from build123d import *

# Parameters (mm, degrees)
F3_W = 25.4
F3_H = 50.8
F5_R = 6.35


with BuildPart() as f4:
    # F4: sweep along a path in F1
    with BuildLine(Plane.XZ) as f4_path:
        Line((4636.6553444, 766.7224442), (5169.5693154, 766.7224442))
        Line((5169.5693154, 766.7224442), (5169.5693154, -249.2775558))
        Line((5169.5693154, -249.2775558), (4636.6553444, -249.2775558))
    # F3 (on plane+point) → F4 (sweep)
    with BuildSketch(Plane.YZ.offset(4636.6553444)):
        with Locations((0, 766.7224442)):
            Rectangle(F3_W, F3_H)
    sweep(path=f4_path.line, transition=Transition.RIGHT)

    # F5
    f5_edges = [f4.edges().sort_by_distance(p)[0] for p in [
        (4890.41233, 12.7, -223.877556),
        (5144.169315, 12.7, 258.722444),
        (5194.969315, 12.7, 258.722444),
        (4915.81233, 12.7, -274.677556),
        (4890.41233, -12.7, -223.877556),
        (5144.169315, -12.7, 258.722444),
        (4890.41233, 12.7, 741.322444),
        (4915.81233, 12.7, 792.122444),
        (4915.81233, -12.7, 792.122444),
        (4890.41233, -12.7, 741.322444),
        (5194.969315, -12.7, 258.722444),
        (4915.81233, -12.7, -274.677556),
    ]]
    fillet(f5_edges, radius=F5_R)


solid = f4.part
Could you check a few things on this model? Use its own coordinates, in mm. Coordinates: 2 decimals unless noted, no trailing zeros. Loops run counter-clockwise (first coordinate to the right, second up) from the corner with the lowest first, then second, coordinate; pieces in that order, holes last.
1. For P1, Ø10, axis at y = -1.5, z = 405, coming from the -X side; P2, Ø1, axis at x = 4915.5, y = -8.5, coming from the +Z side, each with a flat end and sliding along its axis, tell me the tip position at first contact or that it passes through.
2. Imagine slicing it at A-A (x = 5048). Please give me the cut outline in (y, z).
3. I need wall thicknesses on L1, parallel to Z at x = 4903.5, y = -4; L2, parallel to X at y = 4.75, z = 712.5; L3, parallel to Z at x = 5103, y = -10. Which ranges of each line are inside material? Lowest first, please.
4. Imagine slicing it at B-B (z = 382). Please give me the cut outline in (x, y).
Computed values:
1. P1: stops at x = 5144.17
1. P2: stops at z = 791.9
2. outline: (-12.7, -268.33) arc R6.35 ccw to (-6.35, -274.68) - (6.35, -274.68) arc R6.35 ccw to (12.7, -268.33) - (12.7, -230.23) arc R6.35 ccw to (6.35, -223.88) - (-6.35, -223.88) arc R6.35 ccw to (-12.7, -230.23) - close; (-12.7, 747.67) arc R6.35 ccw to (-6.35, 741.32) - (6.35, 741.32) arc R6.35 ccw to (12.7, 747.67) - (12.7, 785.77) arc R6.35 ccw to (6.35, 792.12) - (-6.35, 792.12) arc R6.35 ccw to (-12.7, 785.77) - close
3. L1: z = -274.68 to -223.88, 741.32 to 792.12
3. L2: x = 5144.17 to 5194.97
3. L3: z = -273.52 to -225.03, 742.48 to 790.97
4. outline: (5144.17, -6.35) arc R6.35 ccw to (5150.52, -12.7) - (5188.62, -12.7) arc R6.35 ccw to (5194.97, -6.35) - (5194.97, 6.35) arc R6.35 ccw to (5188.62, 12.7) - (5150.52, 12.7) arc R6.35 ccw to (5144.17, 6.35) - close
